Geometry: final body of the model. Coordinates: model frame, mm. Face numbers are marked on the shaded views. A direction names the side the tool comes from. Round coordinates to 2 decimals unless told otherwise and drop trailing zeros. Loops run counter-clockwise (first coordinate to the right, second up) from the corner with the lowest first, then second, coordinate; pieces in that order, holes last. Notation, with made-up numbers: (-1.5, 19.25) - (18.5, 19.25) arc R23 cw to (18.5, 36.25) - close; hole circle Ø3 at (7.25, 28). An arc over 180 degrees is marked (long way). Return JSON: item names as keys, results as strings. Group by question number.
1. Material intervals for probe 1 along Z at (x, y) = (20, 4.2); probe 2 along Z at (x, y) = (8.5, 6); probe 3 along Z at (x, y) = (-12, 2.25), sorted ascending.
2. Section D-D on x = -12. Return loops of the section in (y, z).
3. Set-up query: the marked faces 1, 2 and 3. Return all of +Z, -Z, +X, -X, +Y, -Y with unobstructed straight access to the full face (end or side cutting, diameter ignored); none if empty.
4. Section B-B on z = -13. Return loops of the section in (x, y), and give its area (3 significant figures).
5. Draft query along X for the marked faces 4, 5, 6 and 7. Return one class per face: +X half, -X half, draft (parallel to the pull), parting line (faces both ways), or undercut.
6. Section A-A on x = 0. Return loops of the section in (y, z), and give its area (3 significant figures).
7. First-contact query: pin 1 Ø1.8 at (x, y) = (16, 4.5) entering from +Z; pin 2 Ø1.5 at (x, z) = (17.5, -11) entering from -Y; pin 3 Ø1 at (x, y) = (8, 6.5) entering from +Z. Flat tips, straight axial feed; report the tip coordinate or a pass-through.
8. Section C-C on z = 0.5. Return loops of the section in (x, y).
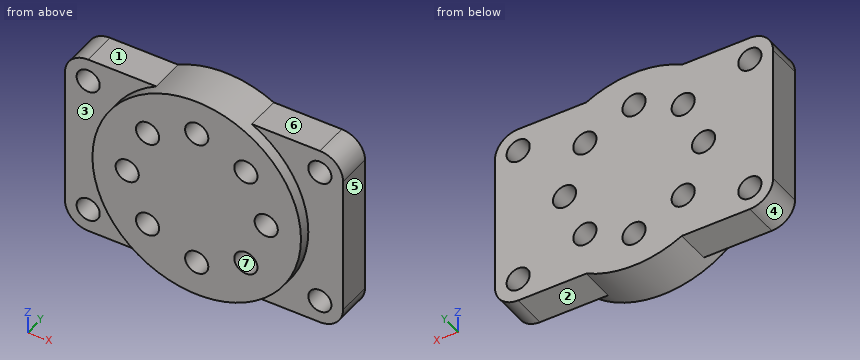
Autodesk Inventor part; units mm, degrees
ref_plane "YZ Plane" through (0, 0, 0) normal (1, 0, 0) x (0, 1, 0)
ref_plane "XZ Plane" through (0, 0, 0) normal (0, 1, 0) x (-1, 0, 0)
ref_plane "XY Plane" through (0, 0, 0) normal (0, 0, 1) x (1, 0, 0)
sketch "Sketch1" plane through (0, 0, 0) normal (0, 1, 0) x (-1, 0, 0)
  circle A0 centre (0, 0) radius 18
  circle A1 centre (0, -12) radius 2
  circle A2 centre (8.4853, -8.4853) radius 2
  circle A3 centre (12, 0) radius 2
  circle A4 centre (8.4853, 8.4853) radius 2
  circle A5 centre (0, 12) radius 2
  circle A6 centre (-8.4853, 8.4853) radius 2
  circle A7 centre (-12, 0) radius 2
  circle A8 centre (-8.4853, -8.4853) radius 2
  dimension "d0" = 36
  dimension "d1" = 4
  dimension "d2" = 12
  dimension "d5" = 360
extrude "Extrusion1" add sketch "Sketch1" along normal blind 8
thread "Thread1"
thread "Thread2"
thread "Thread3"
thread "Thread4"
thread "Thread5"
thread "Thread6"
thread "Thread7"
thread "Thread8"
sketch "Sketch2" plane through (0, 8, 0) normal (0, 1, 0) x (1, 0, 0)
  line L0 (-24, -16) -> (24, -16)
  line L1 (24, -16) -> (24, 16)
  line L2 (24, 16) -> (-24, 16)
  line L3 (-24, 16) -> (-24, -16)
  line L4 (-24, -16) -> (24, 16) construction
  line L5 (24, -16) -> (-24, 16) construction
  circle A0 centre (-20, 12) radius 2
  line L6 (0, 0) -> (0, -16) construction
  line L7 (0, 0) -> (24, 0) construction
  circle A1 centre (0, 0) radius 18
  circle A2 centre (8.4853, 8.4853) radius 2
  circle A3 centre (12, 0) radius 2
  circle A4 centre (8.4853, -8.4853) radius 2
  circle A5 centre (0, -12) radius 2
  circle A6 centre (-8.4853, -8.4853) radius 2
  circle A7 centre (-12, 0) radius 2
  circle A8 centre (-8.4853, 8.4853) radius 2
  circle A9 centre (0, 12) radius 2
  circle A10 centre (20, 12) radius 2
  circle A11 centre (-20, -12) radius 2
  circle A12 centre (20, -12) radius 2
  point P0 (8.2462, 16)
  point P1 (8.2462, -16)
  point P2 (-8.2462, -16)
  point P3 (-8.2462, 16)
  dimension "d25" = 48
  dimension "d26" = 32
  dimension "d27" = 4
  dimension "d28" = 20
  dimension "d29" = 12
extrude "Extrusion2" add sketch "Sketch2" against normal blind 6 contours L3 L2 A1 L0 | A1 L2 L1 L0
fillet "Fillet1" radius 4 4 edges at (-24, 5, 16) (24, 5, 16) (24, 5, -16) (-24, 5, -16)
thread "Thread9"
thread "Thread10"
thread "Thread11"
thread "Thread12"
properties part number "ArmBearingClampingPlate2" material "Aluminum 6061"
Taken from the geometry:
{
 "1": {"probe 1": "-16 to -14, -10 to 10, 14 to 16", "probe 2": "-16 to -10.49, -6.49 to 6.49, 10.49 to 16", "probe 3": "-16 to -2, 2 to 16"},
 "2": {"outline": "(0, -13.42) - (2, -13.42) - (2, -16) - (8, -16) - (8, -2) - (0, -2) - close; (0, 2) - (8, 2) - (8, 16) - (2, 16) - (2, 13.42) - (0, 13.42) - close"},
 "3": {"face 1": "+Z, -X, +Y, -Y", "face 2": "-Z, +X, +Y, -Y", "face 3": "-X, -Y"},
 "4": {"outline": "(-23.87, 2) - (-21.73, 2) - (-21.73, 8) - (-23.87, 8) - close; (-18.27, 2) - (-12.45, 2) - (-12.45, 0) - (-1.73, 0) - (-1.73, 8) - (-18.27, 8) - close; (1.73, 0) - (12.45, 0) - (12.45, 2) - (18.27, 2) - (18.27, 8) - (1.73, 8) - close; (21.73, 2) - (23.87, 2) - (23.87, 8) - (21.73, 8) - close", "area": "267 mm2"},
 "5": {"face 4": "-X half", "face 5": "+X half", "face 6": "draft", "face 7": "undercut"},
 "6": {"outline": "(0, -18) - (8, -18) - (8, -14) - (0, -14) - close; (0, -10) - (8, -10) - (8, 10) - (0, 10) - close; (0, 14) - (8, 14) - (8, 18) - (0, 18) - close", "area": "224 mm2"},
 "7": {"pin 1": "z = 16", "pin 2": "y = 2", "pin 3": "z = 16.36"},
 "8": {"outline": "(-24, 2) - (-17.99, 2) - (-17.99, 0) - (-13.94, 0) - (-13.94, 8) - (-24, 8) - close; (-10.06, 0) - (10.06, 0) - (10.06, 8) - (-10.06, 8) - close; (13.94, 0) - (17.99, 0) - (17.99, 2) - (24, 2) - (24, 8) - (13.94, 8) - close"}
}
